Check sheet for the modelled part. Datum: model origin and axes. Units: mm. A direction names the side the tool comes from. Round coordinates to 2 decimals unless told otherwise and drop trailing zeros. Order: outer loops, then holes, each group sorted by start corner. A loop starts at its lowest first (then second) coordinate and runs counter-clockwise, first axis right, second up.
(1) Sectioned sample at B-B, the plane x = 0. Enter the section's corners in (y, z) (3 decimals), and give its area (3 significant figures).
(2) Sectioned sample at C-C, the plane y = -5.5. Enter the section's corners in (x, z) (3 decimals).
(3) Thickness scan on probe 1 along X at (y, z) = (17.6, 12.7); probe 2 along Y at (x, z) = (3.75, 41.5) (3 decimals); probe 3 along Z at (x, y) = (-6.5, 0) (3 decimals). Record the ranges inside material, lowest first.
(4) Mould release check, pull along Y, two halves, no side actions. Record for faces 1 (the cylindrical face through (-1.57, -16.07, 1.57)), 2 (the flat face through (0, 17, 47.625)), 3 (the cylindrical face through (11.936, -17.691, 1.61)), 4 (the cylindrical face through (-0.18, 16.83, 1.67)): released by +Y, released by -Y, zero draft, split by the parting line, or undercut.
(5) Sectioned sample at A-A, the plane z = 31.75. Enter the section's corners in (x, y) (3 decimals), and give its area (3 significant figures).
(6) Tool access check on faces 5 (the cylindrical face through (0.725, 16.85, 34.052)), 6 (the flat face through (0, 15.24, 26)). Record the directions out of +Z, -Z, +X, -X, +Y, -Y that give a thin tool (end or side, any length) a straight path to the whole face; none if there is none.
(7) Sectioned sample at D-D, the plane y = 14. Enter the section's corners in (x, z).
(8) Depth check by flat-ended pin: pin 1 (12 mm diameter, centred on x = 1, z = 38, fed in from -Y); pin 2 (7.5 mm diameter, centred on x = -5, y = -8.5, fed in from +Z) (3 decimals). Enter the tip coordinate at first touch or a pass-through.
```python
from build123d import *

# Parameters (mm, degrees)
SKETCH1_W              = 25.4
SKETCH1_H              = 36.83
SKETCH1_R              = 2.413
BOSS_EXTRUDE1_DEPTH    = 3.175
SKETCH2_W              = 25.4
SKETCH2_H              = 3.175
BOSS_EXTRUDE2_DEPTH    = 44.45
SKETCH3_R              = 2.413
CUT_EXTRUDE1_DEPTH     = 44.45
FILLET1_R              = 2.54
CONVERT_SOLID1_START   = -12.7
CONVERT_SOLID1_DEPTH   = 25.4
CONVERT_SOLID1_2_DEPTH = 25.4


# Read off the part's stored shape, not the designer's step: Convert-Solid1
with BuildPart() as part:
    # Sketch1 → Boss-Extrude1 (new body)
    with BuildSketch(Plane.XY):
        Rectangle(SKETCH1_W, SKETCH1_H)
        with Locations((0, 4.445)):
            Circle(SKETCH1_R, mode=Mode.SUBTRACT)
        with Locations((0.348627451, -14.605)):
            Circle(SKETCH1_R, mode=Mode.SUBTRACT)
    extrude(amount=BOSS_EXTRUDE1_DEPTH)

    # Sketch2 → Boss-Extrude2 (add)
    with BuildSketch(Plane.XY.offset(3.175)):
        with Locations((0, 16.8275)):
            Rectangle(SKETCH2_W, SKETCH2_H)
    extrude(amount=BOSS_EXTRUDE2_DEPTH)

    # Sketch3 → Cut-Extrude1 (cut)
    with BuildSketch(Plane(origin=(0, 18.415, 0), x_dir=(1, 0, 0), z_dir=(0, 1, 0))):
        with Locations(Location((0, -12.7, 0), (0, 0, 270))):
            Circle(SKETCH3_R)
        with Locations(Location((0, -31.75, 0), (0, 0, 270))):
            Circle(SKETCH3_R)
    extrude(amount=-CUT_EXTRUDE1_DEPTH, mode=Mode.SUBTRACT)

    # Fillet1
    fillet1_edges = [part.edges().sort_by_distance(p)[0] for p in [
        (-12.7, 16.8275, 47.625),
        (12.7, 16.8275, 47.625),
        (12.7, -18.415, 1.5875),
        (-12.7, -18.415, 1.5875),
    ]]
    fillet(fillet1_edges, radius=FILLET1_R)

    # Convert-Solid1 outline → Convert-Solid1 (cut)
    with BuildSketch(Plane.YZ.offset(CONVERT_SOLID1_START)):
        with BuildLine():
            Line((18.415, 0), (18.415, 5.555000066))
            ThreePointArc((18.415, 5.555000066), (16.78797815, 1.62702185), (12.859999934, 0))
            Line((12.859999934, 0), (18.415, 0))
        make_face()
    extrude(amount=CONVERT_SOLID1_DEPTH, mode=Mode.SUBTRACT)

    # Convert-Solid1 2 outline → Convert-Solid1 2 (add)
    with BuildSketch(Plane.YZ.offset(CONVERT_SOLID1_START)):
        with BuildLine():
            Line((15.24, 3.175), (15.24, 5.555000066))
            ThreePointArc((15.24, 5.555000066), (14.54291412, 3.87208588), (12.859999934, 3.175))
            Line((12.859999934, 3.175), (15.24, 3.175))
        make_face()
    extrude(amount=CONVERT_SOLID1_2_DEPTH)


solid = part.part
```
Derived:
1. outline: (-18.415, 0) - (-16.993, 0) - (-16.993, 3.175) - (-18.415, 3.175) - close; (-12.217, 0) - (2.032, 0) - (2.032, 3.175) - (-12.217, 3.175) - close; (6.858, 0) - (12.86, 0) arc R5.555 ccw to (18.415, 5.555) - (18.415, 10.287) - (15.24, 10.287) - (15.24, 5.555) arc R2.38 cw to (12.86, 3.175) - (6.858, 3.175) - close; (15.24, 15.113) - (18.415, 15.113) - (18.415, 29.337) - (15.24, 29.337) - close; (15.24, 34.163) - (18.415, 34.163) - (18.415, 47.625) - (15.24, 47.625) - close
1. area: 192 mm2
2. outline: (-12.7, 0) - (12.7, 0) - (12.7, 3.175) - (-12.7, 3.175) - close
3. probe 1: x = -12.7 to -2.41, 2.41 to 12.7
3. probe 2: y = 15.24 to 18.415
3. probe 3: z = 0 to 3.175
4. face 1: undercut
4. face 2: zero draft
4. face 3: released by -Y
4. face 4: released by +Y
5. outline: (-12.7, 15.24) - (-2.413, 15.24) - (-2.413, 18.415) - (-12.7, 18.415) - close; (2.413, 15.24) - (12.7, 15.24) - (12.7, 18.415) - (2.413, 18.415) - close
5. area: 65.3 mm2
6. face 5: +Y, -Y
6. face 6: +Z, +X, -X, -Y
7. outline: (-12.7, 0.12) - (12.7, 0.12) - (12.7, 3.47) - (-12.7, 3.47) - close
8. pin 1: stops at y = 15.24
8. pin 2: stops at z = 3.175
